```python
from build123d import *

# Parameters (mm, degrees)
F0_R      = 13
F1_DEPTH  = 54
F3_DEPTH  = 30
F4_R      = 23
F5_DEPTH  = 12
F7_DEPTH  = 25
F8_R      = 13
F9_DEPTH  = 13
F10_R     = 11
F11_DEPTH = 9
F12_R     = 13
F13_DEPTH = 8
F14_R     = 13
F15_DEPTH = 25
F17_DEPTH = 14
F18_R     = 9
F19_DEPTH = 5
F20_R     = 6
F21_DEPTH = 53
F23_DEPTH = 50
F25_DEPTH = 32


with BuildPart() as f1:
    # F0 (on Front) → F1 (new body)
    with BuildSketch(Plane.XZ):
        Circle(F0_R)
    extrude(amount=F1_DEPTH)

    # F2 (on face) → F3 (cut)
    with BuildSketch(Plane.XZ.offset(54)):
        with BuildLine():
            Line((-13, 0), (0, 0))
            Line((0, 0), (13, 0))
            ThreePointArc((13, 0), (0, 13), (-13, 0))
        make_face()
    extrude(amount=-F3_DEPTH, mode=Mode.SUBTRACT)

    # F4 (on face) → F5 (join)
    with BuildSketch(Plane(origin=(0, 0, 0), x_dir=(-1, 0, 0), z_dir=(0, 1, 0))):
        Circle(F4_R)
    extrude(amount=F5_DEPTH)

    # F6 (on face) → F7 (cut)
    with BuildSketch(Plane(origin=(0, 12, 0), x_dir=(-1, 0, 0), z_dir=(0, 1, 0))):
        with BuildLine():
            ThreePointArc((0, 20.4449764911), (-3, 17.4449764911), (0, 14.4449764911))
            Line((0, 14.4449764911), (0, 20.4449764911))
        make_face()
        with BuildLine():
            Line((0, 20.4449764911), (0, 14.4449764911))
            ThreePointArc((0, 14.4449764911), (2.1213203436, 15.3236561476), (3, 17.4449764911))
            ThreePointArc((3, 17.4449764911), (2.1213203436, 19.5662968347), (0, 20.4449764911))
        make_face()
        with BuildLine():
            ThreePointArc((3, -17.7103122696), (2.1213203436, -15.5889919261), (0, -14.7103122696))
            Line((0, -14.7103122696), (0, -20.7103122696))
            ThreePointArc((0, -20.7103122696), (2.1213203436, -19.8316326132), (3, -17.7103122696))
        make_face()
        with BuildLine():
            Line((0, -20.7103122696), (0, -14.7103122696))
            ThreePointArc((0, -14.7103122696), (-3, -17.7103122696), (0, -20.7103122696))
        make_face()
        with BuildLine():
            ThreePointArc((-20.7528914064, 0), (-17.7528914064, -3), (-14.7528914064, 0))
            Line((-14.7528914064, 0), (-20.7528914064, 0))
        make_face()
        with BuildLine():
            Line((-20.7528914064, 0), (-14.7528914064, 0))
            ThreePointArc((-14.7528914064, 0), (-17.7528914064, 3), (-20.7528914064, 0))
        make_face()
        with BuildLine():
            ThreePointArc((20.4494218081, 0), (17.4494218081, 3), (14.4494218081, 0))
            Line((14.4494218081, 0), (20.4494218081, 0))
        make_face()
        with BuildLine():
            Line((20.4494218081, 0), (14.4494218081, 0))
            ThreePointArc((14.4494218081, 0), (17.4494218081, -3), (20.4494218081, 0))
        make_face()
    extrude(amount=-F7_DEPTH, mode=Mode.SUBTRACT)

    # F8 (on face) → F9 (join)
    with BuildSketch(Plane(origin=(0, 12, 0), x_dir=(-1, 0, 0), z_dir=(0, 1, 0))):
        Circle(F8_R)
    extrude(amount=F9_DEPTH)

    # F10 (on face) → F11 (join)
    with BuildSketch(Plane(origin=(0, 25, 0), x_dir=(-1, 0, 0), z_dir=(0, 1, 0))):
        Circle(F10_R)
    extrude(amount=F11_DEPTH)

    # F12 (on face) → F13 (join)
    with BuildSketch(Plane(origin=(0, 34, 0), x_dir=(-1, 0, 0), z_dir=(0, 1, 0))):
        Circle(F12_R)
    extrude(amount=F13_DEPTH)

    # F14 (on face) → F15 (join)
    with BuildSketch(Plane(origin=(0, 42, 0), x_dir=(-1, 0, 0), z_dir=(0, 1, 0))):
        Circle(F14_R)
    extrude(amount=F15_DEPTH)

    # F16 (on face) → F17 (cut)
    with BuildSketch(Plane.XY):
        with BuildLine():
            ThreePointArc((0, -45), (2.1213203436, -44.1213203436), (3, -42))
            ThreePointArc((3, -42), (-2.1213203436, -39.8786796564), (0, -45))
        make_face()
    extrude(amount=-F17_DEPTH, mode=Mode.SUBTRACT)

    # F18 (on face) → F19 (join)
    with BuildSketch(Plane(origin=(0, 67, 0), x_dir=(-1, 0, 0), z_dir=(0, 1, 0))):
        Circle(F18_R)
    extrude(amount=F19_DEPTH)

    # F20 (on face) → F21 (join)
    with BuildSketch(Plane(origin=(0, 72, 0), x_dir=(-1, 0, 0), z_dir=(0, 1, 0))):
        Circle(F20_R)
    extrude(amount=F21_DEPTH)

    # F22 (on face) → F23 (cut)
    with BuildSketch(Plane(origin=(0, 125, 0), x_dir=(-1, 0, 0), z_dir=(0, 1, 0))):
        with BuildLine():
            Line((0, 0), (6, 0))
            ThreePointArc((6, 0), (0, 6), (-6, 0))
            Line((-6, 0), (0, 0))
        make_face()
    extrude(amount=-F23_DEPTH, mode=Mode.SUBTRACT)

    # F24 (on face) → F25 (cut)
    with BuildSketch(Plane(origin=(0, 125, 0), x_dir=(-1, 0, 0), z_dir=(0, 1, 0))):
        Polygon((1, 0), (0, 0), (-1, 0), (-1, -7.1843406186), (1, -7.1843406186), align=None)
    extrude(amount=-F25_DEPTH, mode=Mode.SUBTRACT)


solid = f1.part
```
For this review, take the finished solid that the model builds, in its own axes (mm). A direction names the side the tool comes from. Round coordinates to 2 decimals unless told otherwise and drop trailing zeros. Write each loop counter-clockwise with the first axis right and the second up, starting at its lowest first coordinate (ties: lowest second). Pieces come first, ordered by that corner, then holes. Notation, with made-up numbers: (30.5, -21.75) - (57.5, -21.75) arc R37 ccw to (57.5, 16.25) - close; hole circle Ø3 at (-13, 43.5). An arc over 180 degrees is marked (long way). Put each result on its own line as item: value.
Q1. Insertion check: pin 1 Ø9.5 at (x, y) = (0, -42) entering from +Z; pin 2 Ø7 at (x, z) = (17.75, 0) entering from +Y; pin 3 Ø1 at (y, z) = (48.5, 1) entering from +X; pin 4 Ø3.5 at (x, z) = (-17.45, 0) entering from +Y. Each pin has a flat end and moves straight along its axis. Give the tip position at first contact, or say it passes through.
Solved:
pin 1: stops at z = 0
pin 2: stops at y = 12
pin 3: stops at x = 12.99
pin 4: passes through
Q2. Machinability: for faces 4 (the face through (0, 75, 2)), 5 (the face through (1, 109, -3)), 6 (the face through (1.172, 69.465, 8.923)), which of the approach directions +Z, -Z, +X, -X, +Y, -Y give a long, thin tool a straight path to every point of the face, cutting with its end or side? Answer none if there is none.
Solved:
face 4: +Z, +X, -X, +Y
face 5: +Z, -Z, +Y
face 6: +Y
Q3. Wall thickness on probe 1 along Y at (x, z) = (-6, 11); probe 2 along Y at (x, z) = (-14.5, 5.5); probe 3 along Z at (x, y) = (-18, 2): over which ranges is each line inside the solid? List them lowest first.
Solved:
probe 1: y = -24 to 25, 34 to 67
probe 2: y = 0 to 12
probe 3: z = -14.32 to -2.95, 2.95 to 14.32
Q4. We need section D-D (y = 28.5). Give the boundary of the cut face in (x, z), and give its area (3 significant figures).
Solved:
outline: circle Ø22 at (0, 0)
area: 380 mm2
Q5. We need section B-B (y = -36). Give the boundary of the cut face in (x, z).
Solved:
outline: (-13, 0) arc R13 ccw to (13, 0) - close
Q6. We need section C-C (x = 18). Give the boundary of the cut face in (y, z).
Solved:
outline: (0, -14.32) - (12, -14.32) - (12, -2.99) - (0, -2.99) - close; (0, 2.99) - (12, 2.99) - (12, 14.32) - (0, 14.32) - close
Q7. We need section A-A (x = -18.5). Give the boundary of the cut face in (y, z), and give its area (3 significant figures).
Solved:
outline: (0, -13.67) - (12, -13.67) - (12, -2.81) - (0, -2.81) - close; (0, 2.81) - (12, 2.81) - (12, 13.67) - (0, 13.67) - close
area: 261 mm2
Q8. Mouldability with a two-part tool opening along X and no side actions: class faces 1 (the face through (11, 34, 3)), 2 (the face through (-1, 109, -3)), 3 (the face through (2.994, 5.916, 22.804)) as released by +X, released by -X, zero draft, split by the parting line, or undercut.
Solved:
face 1: zero draft
face 2: undercut
face 3: split by the parting line
